Read the model definition and answer for the solid it produces. Units are mm, in the model's axes. A direction names the side the tool comes from. Coordinates: 2 decimals unless noted, no trailing zeros. Loops run counter-clockwise (first coordinate to the right, second up) from the corner with the lowest first, then second, coordinate; pieces in that order, holes last.
Q1. Flat-ended cylindrical pins translate along their axes: P1, Ø2, axis at y = -56, z = 80.5, coming from the -X side; P2, Ø5.5, axis at x = 110, z = 60, coming from the +Y side; P3, Ø10, axis at x = 23.5, z = 82.5, coming from the +Y side; P4, Ø22.5, axis at x = 115, z = 39, coming from the -Y side. Find the tip coordinate at first contact, or state that the pin passes through.
Q2. Section C-C (x = 110) is taken. Give the vertices of the cut face in (y, z), then the cut area to 3 significant figures.
Q3. Section B-B (z = 100) is taken. Give the vertices of the cut face in (x, y), then the cut area to 3 significant figures.
Q4. Section A-A (y = -43.5) is taken. Give the vertices of the cut face in (x, z).
Q5. Section D-D (z = 71) is taken. Give the vertices of the cut face in (x, y).
Q6. Which of the six approach directions +Z, -Z, +X, -X, +Y, -Y give full straight-line access (tool end or side, diameter ignored) to faces 1 (the face through (-107, 0, 59)), 2 (the face through (98, -43, 59)), 3 (the face through (5, -86, 59))?
Q7. The mould has two halves that part along X. Classify faces 4 (the face through (-99.8, 2, 61.1)), 5 (the face through (115, 0, 59)), 6 (the face through (-90, -45, 59)): pulls with the +X half, pulls with the -X half, needs draft (parallel to the pull), parting line crosses it, or undercut.
Q8. Straight lines are drawn through the part: line 1 (Z direction, x = -102, y = 1); line 2 (X direction, y = 1.4, z = 60); line 3 (X direction, y = -78, z = 9). For each, find the intervals that lie inside material, in ascending order.
Autodesk Inventor part; units mm, degrees
ref_plane "YZ Plane" through (0, 0, 0) normal (1, 0, 0) x (0, 1, 0)
ref_plane "XZ Plane" through (0, 0, 0) normal (0, 1, 0) x (-1, 0, 0)
ref_plane "XY Plane" through (0, 0, 0) normal (0, 0, 1) x (1, 0, 0)
sketch "Sketch1" plane through (0, 0, 0) normal (0, 0, 1) x (1, 0, 0)
  line L0 (98, 0) -> (98, -90)
  line L1 (98, -90) -> (-90, -90)
  line L2 (-90, -90) -> (-90, 0)
  line L3 (126, 4) -> (126, 0)
  line L4 (126, 0) -> (-118, 0)
  line L5 (-118, 0) -> (-118, 4)
  line L6 (-86, 4) -> (94, 4)
  line L7 (94, 4) -> (94, -86)
  line L8 (94, -86) -> (-86, -86)
  line L9 (-86, -86) -> (-86, 4)
  line L10 (-90, 0) -> (-86, 0)
  line L11 (94, 0) -> (98, 0)
  line L12 (-118, 4) -> (-86, 4)
  line L13 (94, 4) -> (126, 4)
  point P0 (0, 0)
  point P1 (6, -4)
  point P2 (126, 2)
  point P3 (98, 0)
  dimension "d0" = 188
  dimension "d1" = 90
  dimension "d3" = 90
  dimension "d4" = 244
  dimension "d5" = 120
  dimension "d8" = 90
  dimension "d9" = 180
  dimension "d10" = 4
  dimension "d13" = 0
  dimension "d14" = 4
  dimension "d91" = 32
extrude "Extrusion1" add sketch "Sketch1" along normal blind 120 contours L4 L7 L13 L3 | L0 L1 L2 L4 L9 L8 L7 | L4 L5 L12 L9
fillet "Fillet1" radius 2 4 edges at (-86, -86, 60) (-86, 4, 60) (94, 4, 60) (98, -90, 60)
fillet "Fillet2" radius 2 2 edges at (-90, -90, 60) (94, -86, 60)
sketch "Sketch7" plane through (-118, 4, 120) normal (0, 1, 0) x (1, 0, 0)
  point P0 (118, 120)
sketch "Sketch8" plane through (126, 4, 120) normal (0, 1, 0) x (1, 0, 0)
  line L0 (0, 120) -> (0, 0)
  line L1 (-34, 0) -> (-210, 0)
  line L2 (-244, 120) -> (-244, 0)
  line L3 (-214, 0) -> (-244, 0)
  point P0 (-126, 120)
  point P1 (-16, 100)
  point P2 (-16, 60)
  point P3 (-16, 20)
  point P4 (-228, 100)
  point P5 (-228, 60)
  point P6 (-228, 20)
  dimension "d72" = 16
  dimension "d73" = 16
  dimension "d74" = 16
  dimension "d75" = 20
  dimension "d76" = 40
  dimension "d77" = 40
  dimension "d78" = 16
  dimension "d79" = 40
  dimension "d80" = 40
  dimension "d81" = 20
  dimension "d82" = 16
  dimension "d83" = 16
hole "Hole6" at (110, 4, 20) at (110, 4, 60) at (110, 4, 100) at (-102, 4, 20) at (-102, 4, 60) at (-102, 4, 100) direction (0, -1, 0) diameter 4.917 end through all
equation "\"d89\" = Thickness"
equation "\"BendRadius\" = Thickness"
equation "\"BendReliefWidth\" = Thickness"
equation "\"BendReliefDepth\" = 0.5 * Thickness"
equation "\"CornerReliefSize\" = 4 * Thickness"
equation "\"MinimumRemnant\" = 2 * Thickness"
equation "\"TransitionRadius\" = BendRadius"
equation "\"JacobiRadiusSize\" = BendRadius"
equation "\"GapSize\" = Thickness"
properties part number "Top joint housing back"
Numbers:
1. P1: stops at x = -90
1. P2: stops at y = 4
1. P3: stops at y = -86
1. P4: stops at y = 0
2. outline: (0, 0) - (4, 0) - (4, 17.54) - (0, 17.54) - close; (0, 22.46) - (4, 22.46) - (4, 57.54) - (0, 57.54) - close; (0, 62.46) - (4, 62.46) - (4, 97.54) - (0, 97.54) - close; (0, 102.46) - (4, 102.46) - (4, 120) - (0, 120) - close
2. area: 421 mm2
3. outline: (-118, 0) - (-104.46, 0) - (-104.46, 4) - (-118, 4) - close; (-99.54, 0) - (-90, 0) - (-90, -88) arc R2 ccw to (-88, -90) - (96, -90) arc R2 ccw to (98, -88) - (98, 0) - (107.54, 0) - (107.54, 4) - (96, 4) arc R2 ccw to (94, 2) - (94, -84) arc R2 cw to (92, -86) - (-84, -86) arc R2 cw to (-86, -84) - (-86, 2) arc R2 ccw to (-88, 4) - (-99.54, 4) - close; (112.46, 0) - (126, 0) - (126, 4) - (112.46, 4) - close
3. area: 1,650 mm2
4. outline: (-90, 0) - (-86, 0) - (-86, 120) - (-90, 120) - close; (94, 0) - (98, 0) - (98, 120) - (94, 120) - close
5. outline: (-118, 0) - (-90, 0) - (-90, -88) arc R2 ccw to (-88, -90) - (96, -90) arc R2 ccw to (98, -88) - (98, 0) - (126, 0) - (126, 4) - (96, 4) arc R2 ccw to (94, 2) - (94, -84) arc R2 cw to (92, -86) - (-84, -86) arc R2 cw to (-86, -84) - (-86, 2) arc R2 ccw to (-88, 4) - (-118, 4) - close
6. face 1: +Z, -Z, -X, -Y
6. face 2: +Z, -Z, +X, -Y
6. face 3: +Z, -Z, +Y
7. face 4: undercut
7. face 5: needs draft
7. face 6: pulls with the -X half
8. line 1: z = 0 to 17.54, 22.46 to 57.54, 62.46 to 97.54, 102.46 to 120
8. line 2: x = -118 to -104.46, -99.54 to -86, 94 to 107.54, 112.46 to 126
8. line 3: x = -90 to -86, 94 to 98
